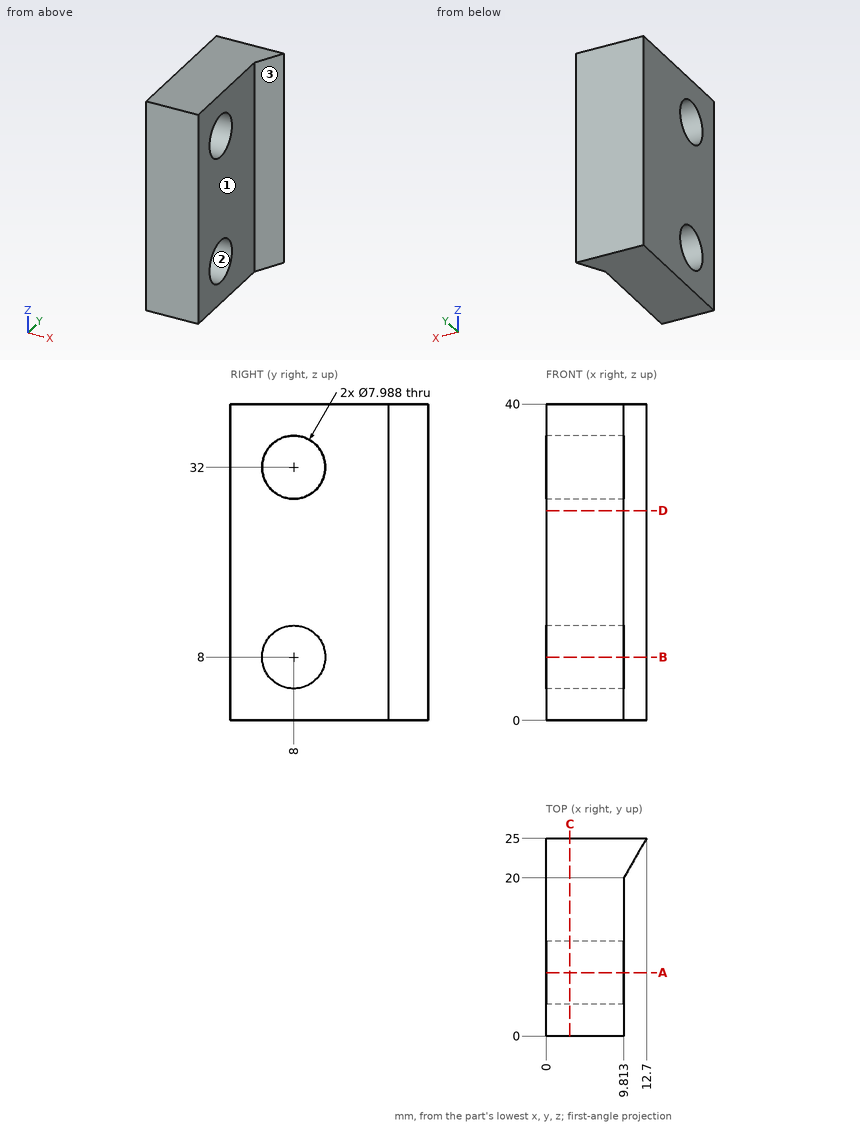
For this review, use the dimensioned drawing (mm, ordinates from the lowest corner) and the shaded views. Give positions to 0.01 mm unless a question says otherwise; leave off trailing zeros. Order: outer loops, then holes, each group sorted by start corner. A loop starts at its lowest first (then second) coordinate and runs counter-clockwise, first axis right, second up. Notation, with made-up numbers: (33.5, 15) -> (57.5, 15) arc R21 ccw to (57.5, 26) -> close; hole circle Ø11 at (68.5, -16.75). An arc over 180 degrees is marked (long way). Write item = value, one per line. Start each with the question number.
(1) Take a section at A-A (y = 8). Write out the cut boundary in (x, z).
(2) Take a section at C-C (x = 3). Write out the cut boundary in (y, z).
(3) Draft analysis for pull direction Y (two halves, no side actions). For the marked faces 1, 2 and 3, state which applies: +Y half, -Y half, draft (parallel to the pull), parting line (faces both ways), or undercut.
(4) Take a section at D-D (z = 26.5). Write out the cut boundary in (x, y), plus the area to 3 significant figures.
(5) For L1, parallel to Y at x = 3.5, z = 32; L2, parallel to Z at x = 1.5, y = 5.75; L3, parallel to Z at x = 7.5, y = 10, list the stretches that pass through material, from the lowest coordinate up. Write a range as from..to.
(6) For pin 1 Ø7 at (y, z) = (8, 32) entering from -X; pin 2 Ø13 at (y, z) = (8, 8) entering from +X, all flat-tipped, find the tip position at first contact; note any pin that passes through.
(7) Take a section at B-B (z = 8). Write out the cut boundary in (x, y).
Returned:
q1.outline = (0, 0) -> (9.81, 0) -> (9.81, 4.01) -> (0, 4.01) -> close; (0, 11.99) -> (9.81, 11.99) -> (9.81, 28.01) -> (0, 28.01) -> close; (0, 35.99) -> (9.81, 35.99) -> (9.81, 40) -> (0, 40) -> close
q2.outline = (0, 0) -> (25, 0) -> (25, 40) -> (0, 40) -> close; hole circle Ø7.99 at (8, 8); hole circle Ø7.99 at (8, 32)
q3.face_1 = draft
q3.face_2 = undercut
q3.face_3 = -Y half
q4.outline = (0, 0) -> (9.81, 0) -> (9.81, 20) -> (12.7, 25) -> (0, 25) -> close
q4.area = 253 mm²
q5.L1 = 0..4.01, 11.99..25
q5.L2 = 0..4.7, 11.3..28.7, 35.3..40
q5.L3 = 0..4.54, 11.46..28.54, 35.46..40
q6.pin_1 = through
q6.pin_2 = 9.81
q7.outline = (0, 0) -> (9.81, 0) -> (9.81, 4.01) -> (0, 4.01) -> close; (0, 11.99) -> (9.81, 11.99) -> (9.81, 20) -> (12.7, 25) -> (0, 25) -> close
